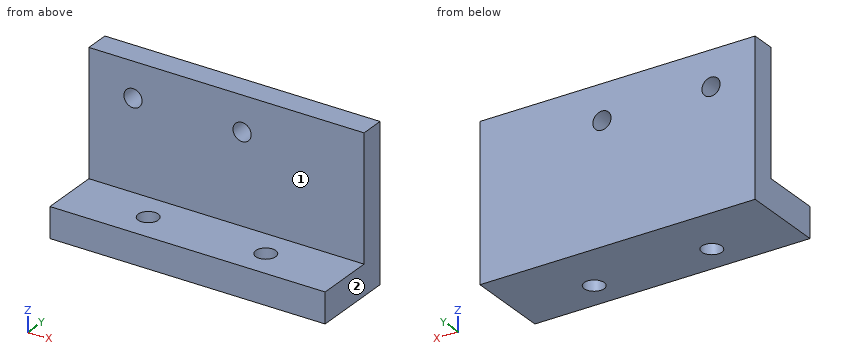
```python
from build123d import *

# Parameters (mm, degrees)
SKETCH1_W           = 45.4
SKETCH1_H           = 25.5
BOSS_EXTRUDE1_DEPTH = 4
SKETCH2_W           = 45.4
SKETCH2_H           = 5
BOSS_EXTRUDE2_DEPTH = 9.75
SKETCH3_R           = 1.5
CUT_EXTRUDE1_DEPTH  = 10
SKETCH7_R           = 1.65
CUT_EXTRUDE3_DEPTH  = 10


with BuildPart() as part:
    # Sketch1 → Boss-Extrude1 (new body)
    with BuildSketch(Plane(origin=(0, 0, 0), x_dir=(1, 0, 0), z_dir=(0, 1, 0))):
        with Locations((22.7, 12.75)):
            Rectangle(SKETCH1_W, SKETCH1_H)
    extrude(amount=BOSS_EXTRUDE1_DEPTH)

    # Sketch2 → Boss-Extrude2 (add)
    with BuildSketch(Plane.XZ):
        with Locations((22.7, -23)):
            Rectangle(SKETCH2_W, SKETCH2_H)
    extrude(amount=BOSS_EXTRUDE2_DEPTH)

    # Sketch3 → Cut-Extrude1 (cut)
    with BuildSketch(Plane(origin=(0, 4, 0), x_dir=(1, 0, 0), z_dir=(0, 1, 0))):
        with Locations((7.278895007, 5.784390941)):
            Circle(SKETCH3_R)
        with Locations((25.277013577, 5.782705683)):
            Circle(SKETCH3_R)
    extrude(amount=-CUT_EXTRUDE1_DEPTH, mode=Mode.SUBTRACT)

    # Sketch7 → Cut-Extrude3 (cut)
    with BuildSketch(Plane.XY.offset(-20.5)):
        with Locations((32.4, -4.881628377)):
            Circle(SKETCH7_R)
        with Locations((13, -4.881628377)):
            Circle(SKETCH7_R)
    extrude(amount=-CUT_EXTRUDE3_DEPTH, mode=Mode.SUBTRACT)


solid = part.part
```
For this review, take the finished solid that the model builds, in its own axes (mm). Face numbers are marked on the shaded views. A direction names the side the tool comes from. Give positions to 0.01 mm unless a question says otherwise; leave off trailing zeros. Order: outer loops, then holes, each group sorted by start corner. A loop starts at its lowest first (then second) coordinate and runs counter-clockwise, first axis right, second up.
1) Insertion check: pin 1 (2 mm diameter, centred on y = -2.5, z = -7.5, fed in from +X); pin 2 (6 mm diameter, centred on x = 30, z = -9.5, fed in from -Y); pin 3 (4 mm diameter, centred on x = 32.4, y = -4.88, fed in from +Z). Each pin has a flat end and moves straight along its axis. Give the tip position at first contact, or say it passes through.
2) Take a section at B-B (y = -6). Give the boundary of the cut face in (x, z).
3) Take a section at A-A (x = 13). Give the boundary of the cut face in (y, z).
4) For the marked faces 1 and 2, list the 3-axis set-ups (+Z, -Z, +X, -X, +Y, -Y) from which the entire face can be reached by the end or side of a thin tool; tool diameter is ignored.
5) Take a section at D-D (z = -1.5). Give the boundary of the cut face in (x, y).
6) Wall thickness on line 1 (Y direction, x = 13, z = -23); line 2 (X direction, y = 3.25, z = -5.5); line 3 (X direction, y = 2.5, z = -6.5): over which ranges is each line inside the solid? List them lowest first.
7) Take a section at C-C (x = 18). Give the boundary of the cut face in (y, z).
Derived:
1. pin 1: passes through
1. pin 2: stops at y = 0
1. pin 3: stops at z = -20.5
2. outline: (0, -25.5) - (11.79, -25.5) - (11.79, -20.5) - (0, -20.5) - close; (14.21, -25.5) - (31.19, -25.5) - (31.19, -20.5) - (14.21, -20.5) - close; (33.61, -25.5) - (45.4, -25.5) - (45.4, -20.5) - (33.61, -20.5) - close
3. outline: (-9.75, -25.5) - (-6.53, -25.5) - (-6.53, -20.5) - (-9.75, -20.5) - close; (-3.23, -25.5) - (4, -25.5) - (4, 0) - (0, 0) - (0, -20.5) - (-3.23, -20.5) - close
4. face 1: +Z, +X, -X, -Y
4. face 2: +Z, -Z, +X, +Y, -Y
5. outline: (0, 0) - (45.4, 0) - (45.4, 4) - (0, 4) - close
6. line 1: y = -9.75 to -6.53, -3.23 to 4
6. line 2: x = 0 to 5.81, 8.75 to 23.8, 26.75 to 45.4
6. line 3: x = 0 to 5.96, 8.6 to 23.96, 26.59 to 45.4
7. outline: (-9.75, -25.5) - (4, -25.5) - (4, 0) - (0, 0) - (0, -20.5) - (-9.75, -20.5) - close
